from build123d import *

# Parameters (mm, degrees)
PAD_DEPTH           = 5
SKETCH002_R         = 1.05
PAD001_DEPTH        = 3
SKETCH003_R         = 3.65
SKETCH003_R_2       = 2.5
PAD002_DEPTH        = 2.5
SKETCH004_R         = 1.5
POCKET_DEPTH        = 1.1
PAD003_DEPTH        = 2
LINEARPATTERN_COUNT = 2
LINEARPATTERN_PITCH = 5


with BuildPart() as part:
    # Sketch → Pad (new body)
    with BuildSketch(Plane.XY):
        Polygon((-30, 10), (30, 10), (40, 0), (30, -10), (-30, -10), (-40, 0), align=None)
    extrude(amount=PAD_DEPTH)

    # Sketch002 → Pad001 (join)
    with BuildSketch(Plane.YZ.offset(15)):
        with BuildLine():
            Line((-5, 4.9), (5, 4.9))
            Line((5, 4.9), (3.635617, 20.223706))
            ThreePointArc((3.635617, 20.223706), (0, 23.55), (-3.635617, 20.223706))
            Line((-5, 4.9), (-3.635617, 20.223706))
        make_face()
        with Locations((0, 19.9)):
            Circle(SKETCH002_R, mode=Mode.SUBTRACT)
    extrude(amount=PAD001_DEPTH)

    # Sketch003 (on DatumPlane) → Pad002 (join)
    with BuildSketch(Plane(origin=(15, 0, 0), x_dir=(0, -1, 0), z_dir=(-1, 0, 0))):
        with Locations((0, 19.9)):
            Circle(SKETCH003_R)
        with Locations((0, 19.9)):
            Circle(SKETCH003_R_2, mode=Mode.SUBTRACT)
    extrude(amount=PAD002_DEPTH)

    # Sketch004 (on DatumPlane) → Pocket (cut)
    with BuildSketch(Plane.YZ.offset(18)):
        with Locations((0, 19.9)):
            Circle(SKETCH004_R)
    extrude(amount=-POCKET_DEPTH, mode=Mode.SUBTRACT)

    # Sketch005 → Pad003 (join)
    with BuildSketch(Plane.XZ.offset(1.5)):
        Polygon((10, 5), (15, 10), (15, 5), align=None)
    pad003 = extrude(amount=PAD003_DEPTH)

    # LinearPattern: Pad003 ×2
    with Locations(*[(0, i * LINEARPATTERN_PITCH, 0) for i in range(1, LINEARPATTERN_COUNT)]):
        add(pad003)


solid = part.part
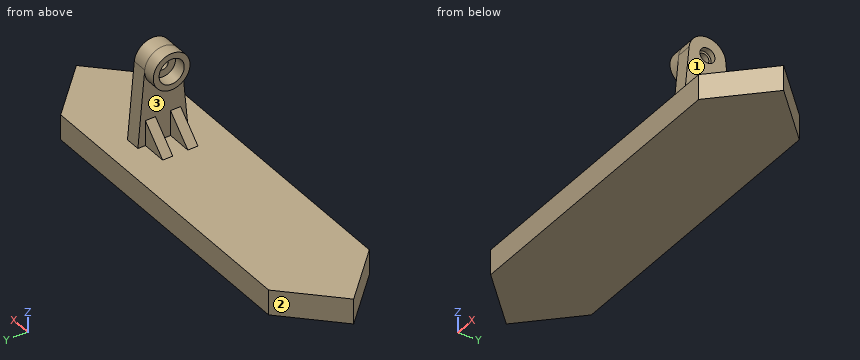
Part model, mm, in its own coordinate system. Face numbers are marked on the shaded views. A direction names the side the tool comes from. Coordinates: 2 decimals unless noted, no trailing zeros. Loops run counter-clockwise (first coordinate to the right, second up) from the corner with the lowest first, then second, coordinate; pieces in that order, holes last. Notation, with made-up numbers: (63, -37) -> (80, -37) arc R10 ccw to (80, -24) -> close; hole circle Ø7 at (21, -6.5). An arc over 180 degrees is marked (long way). Use a Markdown table: item, result. Add a question column.
Item 1: Which spindle directions (+Z, -Z, +X, -X, +Y, -Y) get a long thin tool onto all of the face, cutting with end or side? Do the marked faces 1, 2 and 3. Say none if no direction does.
Item 2: Band-saw the part on B-B on x = 31. Write the cut outline in (y, z).
Item 3: Band-saw the part on C-C on y = 8.75. Write the cut outline in (x, z).
Item 4: Band-saw the part on A-A on z = 8. Write the cut outline in (x, y).
Item 5: Probe probe 1 along Z at (x, y) = (13.25, 0); probe 2 along Y at (x, z) = (16.1, 19.9); probe 3 along Z at (x, y) = (-34, -4). List the from-to ranges inside material, lowest first.
Item 6: Flat gauge pins, fed straight in: P1, Ø2.5, axis at x = 13, z = 7.5, coming from the -Y side; P2, Ø2.5, axis at y = 0, z = 19.9, coming from the -X side; P3, Ø2.5, axis at y = -2.5, z = 22, coming from the +X side; P4, Ø10, axis at y = -3.5, z = 2.5, coming from the -X side. Where does each tip first touch, or does it go through?
Geometry says:
| question | item | result |
|---|---|---|
| 1 | face 1 | +Z, +X, +Y, -Y |
| 1 | face 2 | +Z, -Z, -X, +Y |
| 1 | face 3 | -X |
| 2 | outline | (-9, 0) -> (9, 0) -> (9, 5) -> (-9, 5) -> close |
| 3 | outline | (-31.25, 0) -> (31.25, 0) -> (31.25, 5) -> (-31.25, 5) -> close |
| 4 | outline | (13, -3.5) -> (15, -3.5) -> (15, -4.72) -> (18, -4.72) -> (18, 4.72) -> (15, 4.72) -> (15, 3.5) -> (13, 3.5) -> (13, 1.5) -> (15, 1.5) -> (15, -1.5) -> (13, -1.5) -> close |
| 5 | probe 1 | 0 to 5, 16.25 to 17.4, 22.4 to 23.55 |
| 5 | probe 2 | -3.66 to -1.05, 1.05 to 3.66 |
| 5 | probe 3 | 0 to 5 |
| 6 | P1 | y = -3.5 |
| 6 | P2 | x = 15 |
| 6 | P3 | x = 18 |
| 6 | P4 | x = -40 |
